from build123d import *

# Parameters (mm, degrees)
SKETCH_2_R      = 2.75
EXTRUDE_1_DEPTH = 6
EXTRUDE_2_DEPTH = 6


with BuildPart() as part:
    # По траектории1: sweep along a path in Эскиз1
    with BuildLine(Plane(origin=(0, 0, 0), x_dir=(1, 0, 0), z_dir=(0, 1, 0))) as sweep_1_path:
        Line((0, 0), (0, 10))
        ThreePointArc((0, 10), (2.928932188, 17.071067812), (10, 20))
        Line((10, 20), (59.5, 20))
        ThreePointArc((59.5, 20), (66.571067812, 17.071067812), (69.5, 10))
        Line((69.5, 10), (69.5, 0))
    # Эскиз2 → По траектории1 (sweep)
    with BuildSketch(Plane.XY):
        Circle(SKETCH_2_R)
    sweep(path=sweep_1_path.line)

    # Эскиз3 → Бобышка-Вытянуть1 (add)
    with BuildSketch(Plane.XY):
        Polygon((-6, 3), (6, 3), (7.5, -2.809475019), (-7.5, -2.809475019), align=None)
    extrude(amount=-EXTRUDE_1_DEPTH)

    # Эскиз4 → Бобышка-Вытянуть2 (add)
    with BuildSketch(Plane.XY):
        Polygon((63.5, 3), (75.5, 3), (77, -2.809475019), (62, -2.809475019), align=None)
    extrude(amount=-EXTRUDE_2_DEPTH)


solid = part.part
Design review of the part built by this model. Coordinates are the model's own, in mm. A direction names the side the tool comes from. Give positions to 0.01 mm unless a question says otherwise; leave off trailing zeros. Loops run counter-clockwise (first coordinate to the right, second up) from the corner with the lowest first, then second, coordinate; pieces in that order, holes last. Notation, with made-up numbers: (49, -7) -> (71, -7) arc R32 cw to (71, 30) -> close; hole circle Ø9 at (-36, 72.25). An arc over 180 degrees is marked (long way). One line per question, with ' | ' between items. Start each with the question number.
(1) Draft analysis for pull direction Z (two halves, no side actions). For faces 4 (the face through (-0.596, 2.685, -8.028)), 5 (the face through (35.096, -0.121, -22.747)), 6 (the face through (0, 0, 0)), 7 (the face through (0, 3, -3)), state which applies: +Z half, -Z half, draft (parallel to the pull), parting line (faces both ways), or undercut.
(2) We need section A-A (z = -4.5). State the section outline as (x, y) points, and give its area (3 significant figures).
(3) We need section B-B (y = -2). State the section outline as (x, z) points.
(4) We need section C-C (x = 46). State the section outline as (y, z) points, and give its area (3 significant figures).
(5) We need section D-D (z = -8). State the section outline as (x, y) points.
(6) Insertion check: P1, Ø1.7, axis at x = 68, y = 0, coming from the -Z side; P2, Ø8, axis at x = 25, z = -16, coming from the +Y side. Each pin has a flat end and moves straight along its axis. Give the tip position at first contact, or say it passes through.
(7) For faces 1 (the face through (6.74, 0.14, -2.96)), 2 (the face through (70, -2.809, -3)), 3 (the face through (72.247, -0.121, -7.972)), list the 3-axis set-ups (+Z, -Z, +X, -X, +Y, -Y) from which the entire face can be reached by the end or side of a thin tool; tool diameter is ignored.
(8) For line 1 (X direction, y = -2.3, z = -15); line 2 (X direction, y = -2.1, z = -1.25); line 3 (Z direction, x = 36.5, y = 0.2), list the stretches that pass through material, from the lowest coordinate up.
The answers:
1) face 4: undercut | face 5: parting line | face 6: +Z half | face 7: draft
2) outline: (-7.5, -2.81) -> (7.5, -2.81) -> (6, 3) -> (-6, 3) -> close; (62, -2.81) -> (77, -2.81) -> (75.5, 3) -> (63.5, 3) -> close | area: 157 mm^2
3) outline: (-7.29, -6) -> (-1.89, -6) -> (-1.89, -10) arc R11.89 ccw to (10, -21.89) -> (59.5, -21.89) arc R11.89 ccw to (71.39, -10) -> (71.39, -6) -> (76.79, -6) -> (76.79, 0) -> (62.21, 0) -> (62.21, -6) -> (67.61, -6) -> (67.61, -10) arc R8.11 cw to (59.5, -18.11) -> (10, -18.11) arc R8.11 cw to (1.89, -10) -> (1.89, -6) -> (7.29, -6) -> (7.29, 0) -> (-7.29, 0) -> close
4) outline: circle Ø5.5 at (0, -20) | area: 23.8 mm^2
5) outline: circle Ø5.5 at (0, 0); circle Ø5.5 at (69.5, 0)
6) P1: stops at z = -20.2 | P2: stops at y = 2.75
7) face 1: +Z, +Y | face 2: +Z, -Z, +X, -X, -Y | face 3: none
8) line 1: x = -0.36 to 3.14, 66.36 to 69.86 | line 2: x = -7.32 to 7.32, 62.18 to 76.82 | line 3: z = -22.74 to -17.26
